Can you work these out from the model? Positions are in its coordinate system, mm. Give positions to 0.01 mm unless a question says otherwise; leave off trailing zeros. Write each loop counter-clockwise with the first axis right and the second up, starting at its lowest first coordinate (ties: lowest second). Pieces come first, ordered by that corner, then holes.
Autodesk Inventor part; units mm, degrees
ref_plane "YZ Plane" through (0, 0, 0) normal (1, 0, 0) x (0, 1, 0)
ref_plane "XZ Plane" through (0, 0, 0) normal (0, 1, 0) x (-1, 0, 0)
ref_plane "XY Plane" through (0, 0, 0) normal (0, 0, 1) x (1, 0, 0)
sketch "Sketch1" plane through (0, 0, 0) normal (0, 0, 1) x (1, 0, 0)
  circle A0 centre (0, 0) radius 7.9375
  line L0 (-25.4, 25.4) -> (25.4, 25.4)
  line L1 (25.4, 25.4) -> (25.4, -25.4)
  line L2 (25.4, -25.4) -> (-25.4, -25.4)
  line L3 (-25.4, -25.4) -> (-25.4, 25.4)
  line L4 (-25.4, 25.4) -> (0, 0) construction
  line L5 (0, 0) -> (25.4, 25.4) construction
  line L6 (8.2489, 14.2875) -> (16.4978, 0) construction
  line L7 (16.4978, 0) -> (8.2489, -14.2875) construction
  line L8 (8.2489, -14.2875) -> (-8.2489, -14.2875) construction
  line L9 (-8.2489, -14.2875) -> (-16.4978, 0) construction
  line L10 (-16.4978, 0) -> (-8.2489, 14.2875) construction
  line L11 (-8.2489, 14.2875) -> (8.2489, 14.2875) construction
  circle A1 centre (-8.2489, 14.2875) radius 2.4384
  circle A2 centre (16.4978, 0) radius 2.4384
  circle A3 centre (-8.2489, -14.2875) radius 2.4384
  line L12 (0, 0) -> (-25.4, -25.4) construction
  line L13 (0, 0) -> (25.4, -25.4) construction
  dimension "d0" = 50.8
  dimension "d1" = 28.575
  dimension "d2" = 15.875
  dimension "d3" = 4.8768
extrude "Extrusion1" add sketch "Sketch1" along normal blind 3.175
properties part number "BearingRetainerPlate" material "Aluminum-6061"
1) Suppose I cut it at B-B on x = 0. Write out the boundary of the cut face in (y, z) (1 decimal).
Values follow:
outline: (-25.4, 0) - (-7.9, 0) - (-7.9, 3.2) - (-25.4, 3.2) - close; (7.9, 0) - (25.4, 0) - (25.4, 3.2) - (7.9, 3.2) - close
2) If we mould it in two halves opening along Y, with no side actions, what happens to faces 1 (the face through (-25.4, 0, 2)), 2 (the face through (0, 25.4, 2)), 3 (the face through (-6, -13.35, 1.57))? For each: +Y half, -Y half, draft (parallel to the pull), parting line (faces both ways), or undercut.
Values follow:
face 1: draft
face 2: +Y half
face 3: undercut
3) Suppose I cut it at A-A on y = 0. Write out the boundary of the cut face in (x, z) (1 decimal).
Values follow:
outline: (-25.4, 0) - (-7.9, 0) - (-7.9, 3.2) - (-25.4, 3.2) - close; (7.9, 0) - (14.1, 0) - (14.1, 3.2) - (7.9, 3.2) - close; (18.9, 0) - (25.4, 0) - (25.4, 3.2) - (18.9, 3.2) - close
4) Suppose I cut it at C-C on y = -15. Write out the boundary of the cut face in (x, z) (3 decimals).
Values follow:
outline: (-25.4, 0) - (-10.581, 0) - (-10.581, 3.175) - (-25.4, 3.175) - close; (-5.917, 0) - (25.4, 0) - (25.4, 3.175) - (-5.917, 3.175) - close
5) Please list where these lines run through material, in increasing order: L1, parallel to Y at x = 0, z = 0.6; L2, parallel to X at y = -2.5, z = 0.7; L3, parallel to Y at x = 7, z = 2.4.
Values follow:
L1: y = -25.4 to -7.94, 7.94 to 25.4
L2: x = -25.4 to -7.53, 7.53 to 25.4
L3: y = -25.4 to -3.74, 3.74 to 25.4
6) Suppose I cut it at D-D on x = -9. Write out the boundary of the cut face in (y, z) (3 decimals), plus the area to 3 significant figures.
Values follow:
outline: (-25.4, 0) - (-16.607, 0) - (-16.607, 3.175) - (-25.4, 3.175) - close; (-11.968, 0) - (11.968, 0) - (11.968, 3.175) - (-11.968, 3.175) - close; (16.607, 0) - (25.4, 0) - (25.4, 3.175) - (16.607, 3.175) - close
area: 132 mm2
